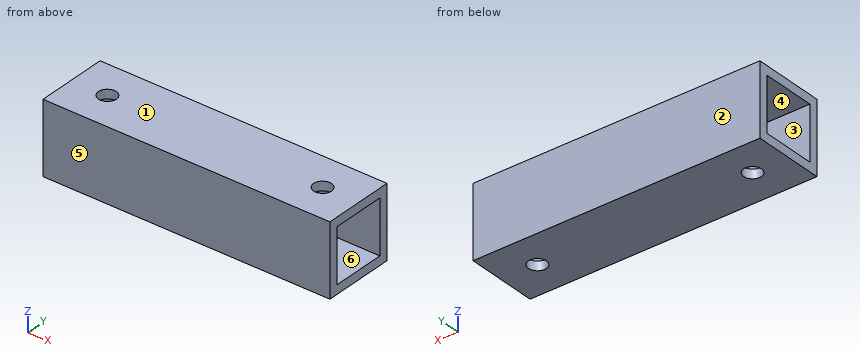
```python
from build123d import *

# Parameters (mm, degrees)
SKETCH1_W           = 101.6
SKETCH1_H           = 25.4
BOSS_EXTRUDE1_DEPTH = 25.4
SKETCH2_W           = 9.525
SKETCH2_H           = 19.040717284
CUT_EXTRUDE1_DEPTH  = 508
SKETCH4_R           = 3.175
CUT_EXTRUDE3_DEPTH  = 508


with BuildPart() as part:
    # Sketch1 → Boss-Extrude1 (new body)
    with BuildSketch(Plane.XY):
        Rectangle(SKETCH1_W, SKETCH1_H)
    extrude(amount=BOSS_EXTRUDE1_DEPTH)

    # Sketch2 → Cut-Extrude1 (cut)
    with BuildSketch(Plane(origin=(50.8, 0, 0), x_dir=(0, 0, -1), z_dir=(1, 0, 0))):
        with Locations((-17.4625, 0)):
            Rectangle(SKETCH2_W, SKETCH2_H)
        with Locations((-7.9375, 0)):
            Rectangle(SKETCH2_W, SKETCH2_H)
    extrude(amount=-CUT_EXTRUDE1_DEPTH, mode=Mode.SUBTRACT)

    # Sketch4 → Cut-Extrude3 (cut)
    with BuildSketch(Plane.XY.offset(25.4)):
        with Locations((-38.1, 0)):
            Circle(SKETCH4_R)
        with Locations((38.1, 0)):
            Circle(SKETCH4_R)
    extrude(amount=-CUT_EXTRUDE3_DEPTH, mode=Mode.SUBTRACT)


solid = part.part
```
Check sheet for the modelled part. Datum: model origin and axes. Units: mm. Face numbers are marked on the shaded views. A direction names the side the tool comes from. Round coordinates to 2 decimals unless told otherwise and drop trailing zeros. Loops run counter-clockwise (first coordinate to the right, second up) from the corner with the lowest first, then second, coordinate; pieces in that order, holes last. Notation, with made-up numbers: (49.5, 72) -> (99.5, 72) arc R21 ccw to (99.5, 86) -> close; hole circle Ø6 at (34.5, 30). An arc over 180 degrees is marked (long way). Answer in a Markdown table with one row per item.
Q1. Thickness scan on L1, parallel to Y at x = -32, z = 15.5; L2, parallel to Z at x = -1, y = -4.5 (3 decimals); L3, parallel to Y at x = -38.1, z = 24 (3 decimals). Record the ranges inside material, lowest first.
Data:
| item | result |
|---|---|
| L1 | y = -12.7 to -9.52, 9.52 to 12.7 |
| L2 | z = 0 to 3.175, 22.225 to 25.4 |
| L3 | y = -12.7 to -3.175, 3.175 to 12.7 |
Q2. Sectioned sample at A-A on y = 0. Enter the section's corners in (x, z) (3 decimals).
Data:
| item | result |
|---|---|
| outline | (-50.8, 0) -> (-41.275, 0) -> (-41.275, 3.175) -> (-50.8, 3.175) -> close; (-50.8, 22.225) -> (-41.275, 22.225) -> (-41.275, 25.4) -> (-50.8, 25.4) -> close; (-34.925, 0) -> (34.925, 0) -> (34.925, 3.175) -> (-34.925, 3.175) -> close; (-34.925, 22.225) -> (34.925, 22.225) -> (34.925, 25.4) -> (-34.925, 25.4) -> close; (41.275, 0) -> (50.8, 0) -> (50.8, 3.175) -> (41.275, 3.175) -> close; (41.275, 22.225) -> (50.8, 22.225) -> (50.8, 25.4) -> (41.275, 25.4) -> close |
Q3. Sectioned sample at D-D on x = -38.1. Enter the section's corners in (y, z) (3 decimals), then the cut area to 3 significant figures.
Data:
| item | result |
|---|---|
| outline | (-12.7, 0) -> (-3.175, 0) -> (-3.175, 3.175) -> (-9.52, 3.175) -> (-9.52, 22.225) -> (-3.175, 22.225) -> (-3.175, 25.4) -> (-12.7, 25.4) -> close; (3.175, 0) -> (12.7, 0) -> (12.7, 25.4) -> (3.175, 25.4) -> (3.175, 22.225) -> (9.52, 22.225) -> (9.52, 3.175) -> (3.175, 3.175) -> close |
| area | 242 mm^2 |
Q4. Sectioned sample at C-C on z = 9.5. Enter the section's corners in (x, y).
Data:
| item | result |
|---|---|
| outline | (-50.8, -12.7) -> (50.8, -12.7) -> (50.8, -9.52) -> (-50.8, -9.52) -> close; (-50.8, 9.52) -> (50.8, 9.52) -> (50.8, 12.7) -> (-50.8, 12.7) -> close |
Q5. Set-up check for the marked faces 5 and 6: record each of +Z, -Z, +X, -X, +Y, -Y from which the full face is reachable in a straight line by a thin tool's end or side.
Data:
| item | result |
|---|---|
| face 5 | +Z, -Z, +X, -X, -Y |
| face 6 | +X, -X |
Q6. Go/stop test with a flat-tipped pin: P1, Ø8, axis at y = 2.5, z = 8, coming from the -X side. Record where the tip stops, or that it passes through.
Data:
| item | result |
|---|---|
| P1 | passes through |
Q7. Sectioned sample at B-B on x = 22. Enter the section's corners in (y, z) (3 decimals).
Data:
| item | result |
|---|---|
| outline | (-12.7, 0) -> (12.7, 0) -> (12.7, 25.4) -> (-12.7, 25.4) -> close; hole (-9.52, 3.175) -> (9.52, 3.175) -> (9.52, 22.225) -> (-9.52, 22.225) -> close |
Q8. Release check for a two-part mould opening along Y. For the marked faces 1, 2, 3 and 4 record: released by +Y, released by -Y, zero draft, split by the parting line, or undercut.
Data:
| item | result |
|---|---|
| face 1 | zero draft |
| face 2 | released by +Y |
| face 3 | undercut |
| face 4 | undercut |
